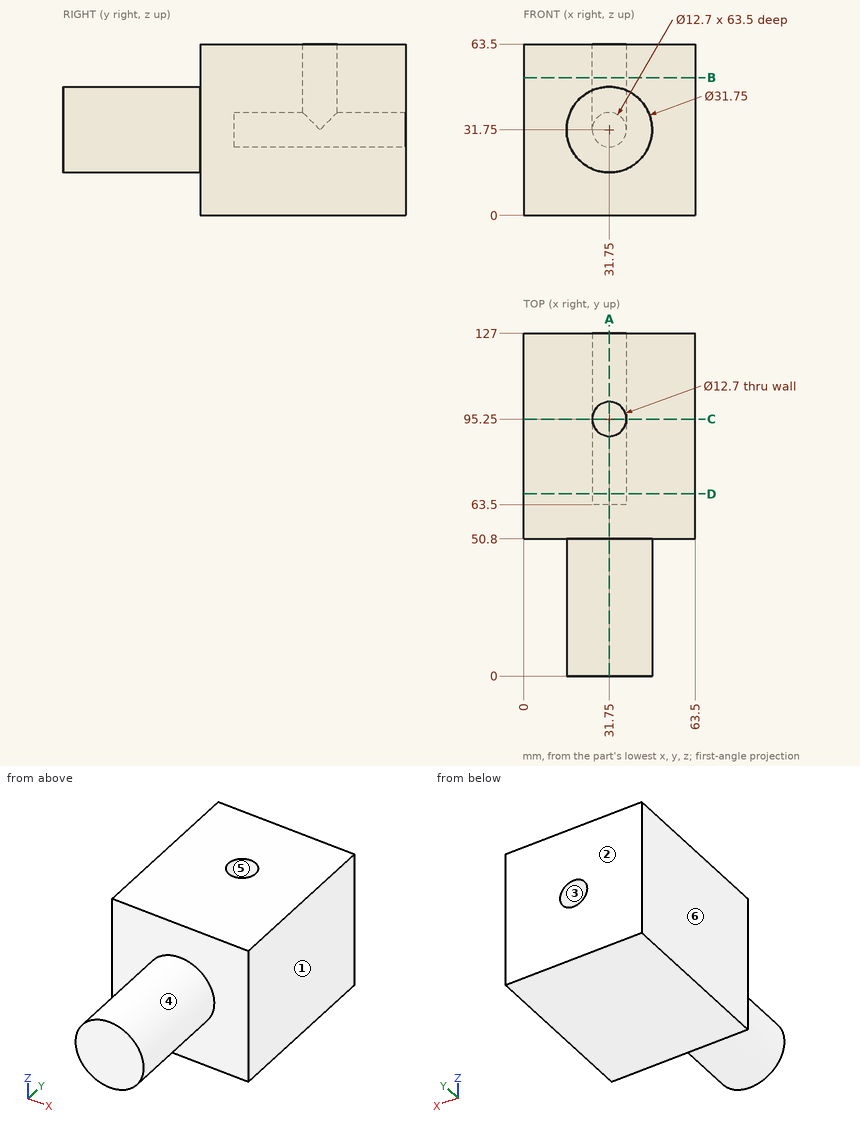
Geometry: see drawing. Coordinates: mm, zero at the bounding-box minimum. A direction names the side the tool comes from. Round coordinates to 2 decimals unless told otherwise and drop trailing zeros. Write each loop counter-clockwise with the first axis right and the second up, starting at its lowest first coordinate (ties: lowest second). Pieces come first, ordered by that corner, then holes. Notation, with made-up numbers: M 87.25,-6.75 L 117.25,-6.75 A20 ccw 117.25,-0.75 Z; hole C 54.25,-12.75 d11. An arc over 180 degrees is marked long. Answer as a JSON object with one key per item and string values. Group by question number.
(1) Section query B-B on z = 51. Output: boundary loops of the cut face in (x, y), then the cut area to 3 significant figures.
(2) Section query D-D on y = 67.5. Output: boundary loops of the cut face in (x, z), then the cut area to 3 significant figures.
(3) First-contact query: pin 1 (6 mm diameter, centred on y = 27.5, z = 44, fed in from +X); pin 2 (8 mm diameter, centred on x = 22, y = 24, fed in from -Z); pin 3 (10 mm diameter, centred on x = 43.5, z = 13, fed in from -Y). Flat tips, straight axial feed; report the tip coordinate or a pass-through.
(4) Ray query, line 1 (Y direction, x = 31.75, z = 57.5); line 2 (Y direction, x = 31.75, z = 43); line 3 (X direction, y = 108, z = 31.75). Return the intervals inside material, ascending. Write a range as [from, to].
(5) Section query A-A on x = 31.75. Output: boundary loops of the cut face in (y, z) (3 decimals), then the cut area to 3 significant figures.
(6) Mould query, pull axis X, two halves, no side actions, for the marked faces 1, 2 and 3. Classes: +X half, -X half, draft (parallel to the pull), parting line (faces both ways), or undercut.
(7) Reachability of the marked faces 4, 5 and 6 from +Z, -Z, +X, -X, +Y, -Y: full face, straight path, thin tool, end or side. Return the list, or none.
(8) Section query C-C on y = 95.25. Output: boundary loops of the cut face in (x, z).
Computed values:
{
 "1": {"outline": "M 0,50.8 L 63.5,50.8 L 63.5,127 L 0,127 Z; hole C 31.75,95.25 d12.7", "area": "4,710 mm^2"},
 "2": {"outline": "M 0,0 L 63.5,0 L 63.5,63.5 L 0,63.5 Z; hole C 31.75,31.75 d12.7", "area": "3,910 mm^2"},
 "3": {"pin 1": "x = 44.65", "pin 2": "z = 16.95", "pin 3": "y = 50.8"},
 "4": {"line 1": "[50.8, 88.9], [101.6, 127]", "line 2": "[0, 88.9], [101.6, 127]", "line 3": "[0, 25.4], [38.1, 63.5]"},
 "5": {"outline": "M 0,15.875 L 50.8,15.875 L 50.8,0 L 127,0 L 127,25.4 L 63.5,25.4 L 63.5,38.1 L 88.9,38.1 L 88.9,63.5 L 50.8,63.5 L 50.8,47.625 L 0,47.625 Z; M 101.6,38.1 L 127,38.1 L 127,63.5 L 101.6,63.5 Z", "area": "5,320 mm^2"},
 "6": {"face 1": "+X half", "face 2": "draft", "face 3": "undercut"},
 "7": {"face 4": "-Y", "face 5": "+Z", "face 6": "+Z, -Z, -X, +Y, -Y"},
 "8": {"outline": "M 0,0 L 63.5,0 L 63.5,63.5 L 38.1,63.5 L 38.1,31.75 A6.35 cw 25.4,31.75 L 25.4,63.5 L 0,63.5 Z"}
}
